For this review, take the finished solid that the model builds, in its own axes (mm). A direction names the side the tool comes from. Give positions to 0.01 mm unless a question says otherwise; leave off trailing zeros. Order: outer loops, then holes, each group sorted by start corner. A loop starts at its lowest first (then second) coordinate and runs counter-clockwise, first axis right, second up. Notation, with made-up numbers: (-38.5, 15) - (16.5, 15) arc R14 cw to (16.5, 29) - close; hole circle Ø8 at (-29.5, 68). An arc over 180 degrees is marked (long way). Answer as a JSON object with one key per item and string values. Group by question number.
from build123d import *

# Parameters (mm, degrees)
BOSS_EXTRUDE1_DEPTH      = 22
SKETCH3_R                = 1.55
CUT_EXTRUDE1_DEPTH       = 30
CUT_EXTRUDE5_DEPTH       = 9
SKETCH11_R               = 1.55
CUT_EXTRUDE10_DEPTH      = 13
CUT_EXTRUDE11_START      = -10
CUT_EXTRUDE11_DEPTH      = 10
SKETCH13_R               = 3
SKETCH13_R_2             = 1.5
CUT_EXTRUDE12_DEPTH      = 72
FILLET1_SIZE             = 7
SKETCH14_W               = 54
SKETCH14_H               = 9.3
SKETCH14_W_2             = 7.05
SKETCH14_H_2             = 4
BOSS_EXTRUDE4_DEPTH      = 4
SKETCH17_W               = 7.05
SKETCH17_H               = 4
BOSS_EXTRUDE5_DEPTH      = 23.05
BOSS_EXTRUDE6_DEPTH      = 27.3
BOSS_EXTRUDE6_DEPTH_BACK = 4
SKETCH18_W               = 54
SKETCH18_H               = 2.95
SKETCH19_W               = 54
SKETCH19_H               = 2.8
BOSS_EXTRUDE7_DEPTH      = 21
FILLET2_SIZE             = 6.5
SKETCH20_R               = 2.625
BOSS_EXTRUDE8_DEPTH      = 6
FILLET4_R                = 1
CUT_EXTRUDE15_DEPTH      = 23.05
SKETCH23_W               = 18.360798368
SKETCH23_H               = 20.1
CUT_EXTRUDE16_DEPTH      = 23
FILLET7_SIZE             = 4
SKETCH26_R               = 1.525
CUT_EXTRUDE18_DEPTH      = 11.5


with BuildPart() as part:
    # Sketch1 → Boss-Extrude1 (new body)
    with BuildSketch(Plane(origin=(0, 0, 0), x_dir=(1, 0, 0), z_dir=(0, 1, 0))):
        Polygon((0, 0), (0, 50), (67, 50), (67, 0), (63, 0), (63, 46), (4, 46), (4, 0), align=None)
    extrude(amount=BOSS_EXTRUDE1_DEPTH)

    # Sketch3 → Cut-Extrude1 (cut)
    with BuildSketch(Plane(origin=(67, 0, 0), x_dir=(0, 0, -1), z_dir=(1, 0, 0))):
        with Locations((12.05, 11)):
            Circle(SKETCH3_R)
    extrude(amount=-CUT_EXTRUDE1_DEPTH, mode=Mode.SUBTRACT)

    # Sketch5 → Cut-Extrude5 (cut)
    with BuildSketch(Plane(origin=(67, 0, 0), x_dir=(0, 0, -1), z_dir=(1, 0, 0))):
        with BuildLine():
            Line((12.05, 22), (0, 22))
            Line((0, 22), (0, 0))
            Line((0, 0), (12.05, 0))
            ThreePointArc((12.05, 0), (1.05, 11), (12.05, 22))
        make_face()
    extrude(amount=-CUT_EXTRUDE5_DEPTH, mode=Mode.SUBTRACT)

    # Sketch11 → Cut-Extrude10 (cut)
    with BuildSketch(Plane(origin=(67, 0, 0), x_dir=(0, 0, -1), z_dir=(1, 0, 0))):
        with Locations((19.05, 11)):
            Circle(SKETCH11_R)
        with Locations((12.05, 18)):
            Circle(SKETCH11_R)
        with Locations((12.05, 4)):
            Circle(SKETCH11_R)
        with Locations((5.05, 11)):
            Circle(SKETCH11_R)
    extrude(amount=-CUT_EXTRUDE10_DEPTH, mode=Mode.SUBTRACT)

    # Sketch12 → Cut-Extrude11 (cut)
    with BuildSketch(Plane.ZY.offset(CUT_EXTRUDE11_START)):
        with BuildLine():
            Line((-12.05, 22), (0, 22))
            Line((0, 22), (0, 0))
            Line((0, 0), (-12.05, 0))
            ThreePointArc((-12.05, 0), (-1.05, 11), (-12.05, 22))
        make_face()
    extrude(amount=CUT_EXTRUDE11_DEPTH, mode=Mode.SUBTRACT)

    # Sketch13 → Cut-Extrude12 (cut)
    with BuildSketch(Plane.ZY):
        with Locations((-12.05, 11)):
            Circle(SKETCH13_R)
        with Locations((-19.05, 11)):
            Circle(SKETCH13_R_2)
        with Locations((-12.05, 4)):
            Circle(SKETCH13_R_2)
        with Locations((-5.05, 11)):
            Circle(SKETCH13_R_2)
        with Locations((-12.05, 18)):
            Circle(SKETCH13_R_2)
    extrude(amount=-CUT_EXTRUDE12_DEPTH, mode=Mode.SUBTRACT)

    # Fillet1
    fillet1_edges = [part.edges().sort_by_distance(p)[0] for p in [
        (63, 11, -46),
        (4, 11, -46),
    ]]
    chamfer(fillet1_edges, length=FILLET1_SIZE)

    # Sketch14 → Boss-Extrude4 (add)
    with BuildSketch(Plane(origin=(0, 0, -50), x_dir=(-1, 0, 0), z_dir=(0, 0, -1))):
        with Locations((-33.5, -4.65)):
            Rectangle(SKETCH14_W, SKETCH14_H)
        with Locations((-56.975, 20)):
            Rectangle(SKETCH14_W_2, SKETCH14_H_2)
        with Locations((-10.025, 20)):
            Rectangle(SKETCH14_W_2, SKETCH14_H_2)
    extrude(amount=-BOSS_EXTRUDE4_DEPTH)

    # Sketch17 → Boss-Extrude5 (add)
    with BuildSketch(Plane(origin=(0, 0, -50), x_dir=(-1, 0, 0), z_dir=(0, 0, -1))):
        with Locations((-56.975, 20)):
            Rectangle(SKETCH17_W, SKETCH17_H)
        with Locations((-10.025, 20)):
            Rectangle(SKETCH17_W, SKETCH17_H)
    extrude(amount=BOSS_EXTRUDE5_DEPTH)

    # Sketch18 → Boss-Extrude6 (add, two sides: drawn at the far end of the back side and taken through both)
    with BuildSketch(Plane.XZ.offset(-18).offset(-BOSS_EXTRUDE6_DEPTH_BACK)):
        with Locations((33.5, -71.575)):
            Rectangle(SKETCH18_W, SKETCH18_H)
    extrude(amount=BOSS_EXTRUDE6_DEPTH + BOSS_EXTRUDE6_DEPTH_BACK)

    # Sketch19 → Boss-Extrude7 (add)
    with BuildSketch(Plane(origin=(0, 0, -50), x_dir=(-1, 0, 0), z_dir=(0, 0, -1))):
        with Locations((-33.5, -7.9)):
            Rectangle(SKETCH19_W, SKETCH19_H)
    extrude(amount=BOSS_EXTRUDE7_DEPTH)

    # Fillet2
    fillet2_edges = [part.edges().sort_by_distance(p)[0] for p in [
        (60.5, 20, -50),
        (6.5, 20, -50),
    ]]
    chamfer(fillet2_edges, length=FILLET2_SIZE - 0.0001)  # a hair under: the kernel refuses the full size

    # Sketch20 → Boss-Extrude8 (add)
    with BuildSketch(Plane.XZ.offset(9.3)):
        with Locations(Location((23.4, -59.65, 0), (0, 0, 270))):
            Circle(SKETCH20_R)
    extrude(amount=BOSS_EXTRUDE8_DEPTH)

    # Fillet4
    fillet4_edges = [part.edges().sort_by_distance(p)[0] for p in [
        (23.4, -15.3, -57.025),
    ]]
    fillet(fillet4_edges, radius=FILLET4_R)

    # Sketch22 → Cut-Extrude15 (cut)
    with BuildSketch(Plane(origin=(0, 0, -73.05), x_dir=(-1, 0, 0), z_dir=(0, 0, -1))):
        Polygon((-60.5, -9.3), (-33.5, -9.3), (-60.5, 18), align=None)
    extrude(amount=-CUT_EXTRUDE15_DEPTH, mode=Mode.SUBTRACT)

    # Sketch23 → Cut-Extrude16 (cut)
    with BuildSketch(Plane(origin=(0, 22, 0), x_dir=(1, 0, 0), z_dir=(0, 1, 0))):
        with Locations((4.369600816, 60.05)):
            Rectangle(SKETCH23_W, SKETCH23_H)
    extrude(amount=-CUT_EXTRUDE16_DEPTH, mode=Mode.SUBTRACT)

    # Fillet7
    fillet7_edges = [part.edges().sort_by_distance(p)[0] for p in [
        (6.5, 0, -48),
    ]]
    chamfer(fillet7_edges, length=FILLET7_SIZE)

    # Sketch26 → Cut-Extrude18 (cut)
    with BuildSketch(Plane(origin=(0, 22, 0), x_dir=(1, 0, 0), z_dir=(0, 1, 0))):
        with Locations(Location((58.21, 64.77, 0), (0, 0, 270))):
            Circle(SKETCH26_R)
        with Locations(Location((58.21, 54.92, 0), (0, 0, 270))):
            Circle(SKETCH26_R)
    extrude(amount=-CUT_EXTRUDE18_DEPTH, mode=Mode.SUBTRACT)


solid = part.part
1) Consider section A-A (z = -64.77). Give the boundary of the cut face in (x, y) (3 decimals).
2) Consider section B-B (z = -44.5). Give the boundary of the cut face in (x, y).
3) For faces 1 (the face through (22, -6.5, -60)), 2 (the face through (27, 10, -73.05)), 3 (the face through (53.45, 20, -60)), list the 3-axis set-ups (+Z, -Z, +X, -X, +Y, -Y) from which the entire face can be reached by the end or side of a thin tool; tool diameter is ignored.
4) Mouldability with a two-part tool opening along X and no side actions: class faces 4 (the face through (60, 11, -42)), 5 (the face through (41.937, -0.769, -70.97)), 6 (the face through (65.028, 19.537, -11.848)) as released by +X, released by -X, zero draft, split by the parting line, or undercut.
5) Consider section D-D (z = -19.05). Give the boundary of the cut face in (x, y).
6) Consider section C-C (x = 48). Give the boundary of the cut face in (y, z).
7) For pin 1 (6 mm diameter, centred on x = 36.5, y = -4, fed in from +Z); pin 2 (5 mm diameter, centred on y = 11, z = -12.05, fed in from -X); pin 3 (12 mm diameter, centred on x = 23, z = -50, fed in from -Y); pin 4 (15 mm diameter, centred on x = 60.5, z = -62, fed in from -Y), all flat-tipped, find the tip position at first contact; note any pin that passes through.
8) For line 1 (Y direction, x = 65.1, z = -12.05); line 2 (Y direction, x = 66, z = -19); line 3 (X direction, y = 20.4, z = -64.77) (3 decimals), list the stretches that pass through material, from the lowest coordinate up.
Result set:
{
 "1": {"outline": "(6.5, -9.3) - (33.5, -9.3) - (36.269, -6.5) - (6.5, -6.5) - close; (53.45, 18) - (56.685, 18) - (56.685, 22) - (53.45, 22) - close; (59.735, 18) - (60.5, 18) - (60.5, 22) - (59.735, 22) - close"},
 "2": {"outline": "(0, 0) - (9.5, 0) - (9.5, 22) - (0, 22) - close; (57.5, 0) - (67, 0) - (67, 22) - (57.5, 22) - close"},
 "3": {"face 1": "+X, -X, +Y", "face 2": "-Z, +X, -X, +Y, -Y", "face 3": "-X, +Y, -Y"},
 "4": {"face 4": "undercut", "face 5": "released by +X", "face 6": "zero draft"},
 "5": {"outline": "(0, 0) - (4, 0) - (4, 9.5) - (0, 9.5) - close; (0, 12.5) - (4, 12.5) - (4, 22) - (0, 22) - close; (63, 0) - (67, 0) - (67, 9.45) - (63, 9.45) - close; (63, 12.55) - (67, 12.55) - (67, 22) - (63, 22) - close"},
 "6": {"outline": "(-9.3, -50) - (22, -50) - (22, -46) - (-9.3, -46) - close; (5.36, -73.05) - (22, -73.05) - (22, -70.1) - (5.36, -70.1) - close"},
 "7": {"pin 1": "stops at z = -46", "pin 2": "passes through", "pin 3": "stops at y = -9.3", "pin 4": "stops at y = 18"},
 "8": {"line 1": "y = 0 to 2.45, 5.55 to 8, 14 to 16.45, 19.55 to 22", "line 2": "y = 0 to 9.45, 12.55 to 22", "line 3": "x = 53.45 to 56.685, 59.735 to 60.5"}
}
